Read the model definition and answer for the solid it produces. Units are mm, in the model's axes. A direction names the side the tool comes from. Round coordinates to 2 decimals unless told otherwise and drop trailing zeros. Write each loop counter-clockwise with the first axis right and the second up, starting at its lowest first coordinate (ties: lowest second). Pieces come first, ordered by that corner, then holes. Notation, with made-up numbers: (39, 31.5) - (77, 31.5) arc R38 ccw to (77, 69.5) - close; hole circle Ø9 at (12, 1). An arc over 180 degrees is marked (long way). One line per item, written item: value. Start each with the question number.
(1) A cutting plane is placed at D-D, the plane y = -5.75. Determine the outline of the cut face in (x, z).
(2) A cutting plane is placed at C-C, the plane z = 6.5. Determine the outline of the cut face in (x, y) (3 decimals), plus the area to 3 significant figures.
(3) Find the intervals of material crossed by L1, parallel to Y at x = 0, z = -1.1 (3 decimals); L2, parallel to Z at x = -5, y = -9.5; L3, parallel to Z at x = 1.75, y = -5.5, in increasing order.
(4) For faces 5 (the face through (0, 9, -5)), 6 (the face through (0, 0, 12.8)), 7 (the face through (5, -5, -53.2)), determine the directions among +Z, -Z, +X, -X, +Y, -Y from which every point of the face is accessible in a straight line to the end or side of a thin tool.
(5) A cutting plane is placed at B-B, the plane y = 0. Determine the outline of the cut face in (x, z) (3 decimals), plus the area to 3 significant figures.
(6) The mould has two halves that part along X. Classify faces 1 (the face through (-0.753, -3.392, 6.31)), 2 (the face through (3, -3, 0)), 3 (the face through (0.77, 9.7, -2.46)), 4 (the face through (-0.186, -7.087, -2.465)): +X half, -X half, draft (parallel to the pull), parting line (faces both ways), or undercut.
(7) A cutting plane is placed at A-A, the plane x = 0. Determine the outline of the cut face in (y, z) (3 decimals), plus the area to 3 significant figures.
(8) Flat-ended cylindrical pins translate along their axes: pin 1 Ø1.5 at (x, y) = (9, 6.5) entering from +Z; pin 2 Ø10 at (x, z) = (-6.5, -14.5) entering from -Y; pin 3 Ø6 at (x, y) = (-10, -2.5) entering from -Z. Find the tip coordinate at first contact, or state that the pin passes through.
from build123d import *

# Parameters (mm, degrees)
SKETCH1_R           = 12.4
BOSS_EXTRUDE1_DEPTH = 53.2
SKETCH2_R           = 3.475
BOSS_EXTRUDE2_DEPTH = 12.8
SKETCH3_R           = 1.425
CUT_EXTRUDE1_DEPTH  = 5
SKETCH4_R           = 6.7
BOSS_EXTRUDE3_DEPTH = 6.7


with BuildPart() as part:
    # Sketch1 → Boss-Extrude1 (new body)
    with BuildSketch(Plane.XY):
        Circle(SKETCH1_R)
    extrude(amount=-BOSS_EXTRUDE1_DEPTH)

    # Sketch2 → Boss-Extrude2 (add)
    with BuildSketch(Plane.XY):
        Circle(SKETCH2_R)
    extrude(amount=BOSS_EXTRUDE2_DEPTH)

    # Sketch3 → Cut-Extrude1 (cut)
    with BuildSketch(Plane.XY):
        with Locations((0, 8.5)):
            Circle(SKETCH3_R)
        with Locations((0, -8.5)):
            Circle(SKETCH3_R)
    extrude(amount=-CUT_EXTRUDE1_DEPTH, mode=Mode.SUBTRACT)

    # Sketch4 → Boss-Extrude3 (add)
    with BuildSketch(Plane(origin=(0, 0, -53.2), x_dir=(-1, 0, 0), z_dir=(0, 0, -1))):
        Circle(SKETCH4_R)
    extrude(amount=BOSS_EXTRUDE3_DEPTH)


solid = part.part
Here are the results:
1. outline: (-10.99, -53.2) - (-3.44, -53.2) - (-3.44, -59.9) - (3.44, -59.9) - (3.44, -53.2) - (10.99, -53.2) - (10.99, 0) - (-10.99, 0) - close
2. outline: circle Ø6.95 at (0, 0)
2. area: 37.9 mm²
3. L1: -12.4 to -9.925, -7.075 to 7.075, 9.925 to 12.4
3. L2: -53.2 to 0
3. L3: -59.9 to 0
4. face 5: +Z
4. face 6: +Z, +X, -X, +Y, -Y
4. face 7: -Z
5. outline: (-12.4, -53.2) - (-6.7, -53.2) - (-6.7, -59.9) - (6.7, -59.9) - (6.7, -53.2) - (12.4, -53.2) - (12.4, 0) - (3.475, 0) - (3.475, 12.8) - (-3.475, 12.8) - (-3.475, 0) - (-12.4, 0) - close
5. area: 1,500 mm²
6. face 1: parting line
6. face 2: draft
6. face 3: undercut
6. face 4: undercut
7. outline: (-12.4, -53.2) - (-6.7, -53.2) - (-6.7, -59.9) - (6.7, -59.9) - (6.7, -53.2) - (12.4, -53.2) - (12.4, 0) - (9.925, 0) - (9.925, -5) - (7.075, -5) - (7.075, 0) - (3.475, 0) - (3.475, 12.8) - (-3.475, 12.8) - (-3.475, 0) - (-7.075, 0) - (-7.075, -5) - (-9.925, -5) - (-9.925, 0) - (-12.4, 0) - close
7. area: 1,470 mm²
8. pin 1: z = 0
8. pin 2: y = -12.31
8. pin 3: z = -53.2
